Autodesk Inventor part; units mm, degrees
ref_plane "YZ Plane" through (0, 0, 0) normal (1, 0, 0) x (0, 1, 0)
ref_plane "XZ Plane" through (0, 0, 0) normal (0, 1, 0) x (-1, 0, 0)
ref_plane "XY Plane" through (0, 0, 0) normal (0, 0, 1) x (1, 0, 0)
sketch "Sketch1" plane through (0, 0, 0) normal (0, 0, 1) x (1, 0, 0)
  arc A0 (-13.2818, 11.9603) -> (-0.6453, -3.2505) centre (-9.7741, 2.02) ccw
  line L0 (-9.7741, 2.02) -> (-0.6453, 7.2905) construction
  line L1 (-9.7741, 2.02) -> (0.7669, 2.02) construction
  line L2 (-9.7741, 2.02) -> (-0.6453, -3.2505) construction
  line L3 (-9.7741, 2.02) -> (0.7669, 2.02) construction
  line L4 (8.2613, 16.5876) -> (8.2613, -12.065) construction
  line L5 (-13.2818, 11.9603) -> (-14.0002, 13.9962)
  arc A1 (-13.2818, 11.9603) -> (0.5715, 0) centre (-9.7741, 2.02) ccw
  line L6 (0.5715, 0) -> (2.7642, 0)
  arc A2 (17.168, -3.2505) -> (29.8044, 11.9603) centre (26.2967, 2.02) ccw
  line L7 (29.8044, 11.9603) -> (30.5229, 13.9962)
  arc A3 (15.9511, 0) -> (29.8044, 11.9603) centre (26.2967, 2.02) ccw
  line L8 (15.9511, 0) -> (13.7584, 0)
  line L9 (-17.9133, -7.729) -> (-17.9133, -30.6279)
  line L10 (-17.9133, -30.6279) -> (-1.615, -30.6279)
  line L11 (-1.615, -30.6279) -> (-1.615, -7.7124)
  line L12 (34.436, -7.729) -> (34.436, -30.6279)
  line L13 (34.436, -30.6279) -> (18.1376, -30.6279)
  line L14 (18.1376, -30.6279) -> (18.1376, -7.7124)
  arc A4 (13.7584, 0) -> (18.1376, -7.7124) centre (26.2967, 2.02) ccw
  arc A5 (34.436, -7.729) -> (30.5229, 13.9962) centre (26.2967, 2.02) ccw
  arc A6 (15.2982, -4.33) -> (18.1376, -7.7124) centre (26.2967, 2.02) ccw
  arc A7 (34.436, -7.729) -> (30.5229, 13.9962) centre (26.2967, 2.02) ccw
  arc A8 (-14.0002, 13.9962) -> (-17.9133, -7.729) centre (-9.7741, 2.02) ccw
  arc A9 (-1.615, -7.7124) -> (1.2244, -4.33) centre (-9.7741, 2.02) ccw
  arc A10 (-14.0002, 13.9962) -> (-17.9133, -7.729) centre (-9.7741, 2.02) ccw
  arc A11 (-1.615, -7.7124) -> (2.7642, 0) centre (-9.7741, 2.02) ccw
  point P0 (0, 0)
  dimension "d0" = 21.082
  dimension "d2" = 30
  dimension "d3" = 30
extrude "Extrusion1" add sketch "Sketch1" along normal blind 50.8
sketch "Sketch2" plane through (-17.9133, -30.6279, 0) normal (0, -1, 0) x (1, 0, 0)
  line L0 (-24.7177, 50.8) -> (77.3849, 50.8)
  line L1 (77.3849, 50.8) -> (77.3849, 0)
  line L2 (77.3849, 0) -> (-24.7177, 0)
  line L3 (-24.7177, 0) -> (-24.7177, 50.8)
  point P0 (17.9133, 0)
extrude "Extrusion2" add sketch "Sketch2" along normal blind 12.7
sketch "Sketch3" plane through (-17.9133, -30.6279, 0) normal (0, 1, 0) x (1, 0, 0)
  point P0 (17.9133, 0)
sketch "Sketch4" plane through (-17.9133, -30.6279, 0) normal (0, 1, 0) x (1, 0, 0)
  point P0 (17.9133, 0)
hole "Hole1" at (49.2151, -30.6279, 40.9398) direction (0, -1, 0) diameter 3.556 end through all countersink diameter 9.525 countersink angle 82
hole "Hole2" at (49.7086, -30.6279, 8.5342) direction (0, -1, 0) diameter 3.556 end through all countersink diameter 9.525 countersink angle 82
hole "Hole3" at (-32.3747, -30.6279, 40.9398) direction (0, -1, 0) diameter 3.556 end through all countersink diameter 9.525 countersink angle 82
hole "Hole4" at (-32.2102, -30.6279, 8.5342) direction (0, -1, 0) diameter 3.556 end through all countersink diameter 9.525 countersink angle 82
thread "Thread1"
thread "Thread2"
thread "Thread3"
thread "Thread4"
thread "Thread5"
thread "Thread6"
Geometry check sheet. Reference: the model listing, model coordinates, mm. A direction names the side the tool comes from. Round coordinates to 2 decimals unless told otherwise and drop trailing zeros. Order: outer loops, then holes, each group sorted by start corner. A loop starts at its lowest first (then second) coordinate and runs counter-clockwise, first axis right, second up. Notation, with made-up numbers: M 13.25,-32 L 72.25,-32 A5 ccw 72.25,-24 Z; hole C 38,40.25 d11. An arc over 180 degrees is marked long. Answer in a Markdown table with one row per item.
(1) Sectioned sample at A-A, the plane y = -18. Record the cut outline in (x, z) (3 decimals).
Responses:
| item | result |
|---|---|
| outline | M -17.913,0 L -1.615,0 L -1.615,50.8 L -17.913,50.8 Z; M 18.138,0 L 34.436,0 L 34.436,50.8 L 18.138,50.8 Z |
(2) Sectioned sample at B-B, the plane y = -6.5. Record the cut outline in (x, z), and give its area (3 significant figures).
Responses:
| item | result |
|---|---|
| outline | M -19.19,0 L -15.98,0 L -15.98,50.8 L -19.19,50.8 Z; M -3.57,0 L -0.36,0 L -0.36,50.8 L -3.57,50.8 Z; M 16.88,0 L 20.09,0 L 20.09,50.8 L 16.88,50.8 Z; M 32.5,0 L 35.71,0 L 35.71,50.8 L 32.5,50.8 Z |
| area | 653 mm² |
(3) Draft check along X on faces 4 (the face through (59.472, -37, 26)), 5 (the face through (-13.636, 12.964, 25.044)), 6 (the face through (-30, -30.628, 26)). Enter one of: released by +X, released by -X, zero draft, split by the parting line, or undercut.
Responses:
| item | result |
|---|---|
| face 4 | released by +X |
| face 5 | undercut |
| face 6 | zero draft |
(4) Sectioned sample at D-D, the plane z = 47. Record the cut outline in (x, y) (1 decimal), and give its area (3 significant figures).
Responses:
| item | result |
|---|---|
| outline | M -42.6,-43.3 L 59.5,-43.3 L 59.5,-30.6 L 34.4,-30.6 L 34.4,-7.7 A12.7 ccw 30.5,14 L 29.8,12 A10.5 cw long 17.2,-3.3 A10.5 cw 16,0 L 13.8,0 A12.7 ccw 18.1,-7.7 L 18.1,-30.6 L -1.6,-30.6 L -1.6,-7.7 A12.7 ccw 1.2,-4.3 A12.7 ccw 2.8,0 L 0.6,0 A10.5 cw -0.6,-3.3 A10.5 cw long -13.3,12 L -14,14 A12.7 ccw -17.9,-7.7 L -17.9,-30.6 L -42.6,-30.6 Z |
| area | 2,190 mm² |
(5) Go/stop test with flat-tipped pins: P1, Ø3, axis at x = -32.21, z = 8.53, coming from the -Y side; P2, Ø10, axis at y = -17.5, z = 38, coming from the +X side; P3, Ø21.5, axis at x = 13, z = 33.5, coming from the +Y side; P4, Ø18.5, axis at y = -15, z = 22.5, coming from the +X side. Record where each tip stops, or that it passes through.
Responses:
| item | result |
|---|---|
| P1 | passes through |
| P2 | stops at x = 34.44 |
| P3 | stops at y = 0 |
| P4 | stops at x = 36.34 |
(6) Sectioned sample at C-C, the plane x = 5. Record the cut outline in (y, z), and give its area (3 significant figures).
Responses:
| item | result |
|---|---|
| outline | M -43.33,0 L -30.63,0 L -30.63,50.8 L -43.33,50.8 Z |
| area | 645 mm² |
(7) Tool access check on faces 1 (the face through (-22.305, 4.087, 25.044)), 2 (the face through (8, -30.628, 26)), 3 (the face through (16.433, -1.699, 25.044)). Record the directions out of +Z, -Z, +X, -X, +Y, -Y that give a thin tool (end or side, any length) a straight path to the whole face; none if there is none.
Responses:
| item | result |
|---|---|
| face 1 | +Z, -Z, -X |
| face 2 | +Z, -Z |
| face 3 | +Z, -Z, +Y |
(8) Scan lines: probe 1 along X at (y, z) = (-9, 41) (3 decimals); probe 2 along X at (y, z) = (-4.5, 27.5); probe 3 along X at (y, z) = (-32, 6.5). Record each from-to range of solid material in increasing order. Write a range as from..to.
Responses:
| item | result |
|---|---|
| probe 1 | x = -17.913..-1.615, 18.138..34.436 |
| probe 2 | x = -20.67..-18.06, -1.49..1.12, 15.4..18.01, 34.58..37.2 |
| probe 3 | x = -42.63..-35.14, -29.28..46.78, 52.64..59.47 |
